Model file for the job. Use its own axes, mm. Face numbers are marked on the shaded views. Coordinates: 2 decimals unless noted, no trailing zeros. Order: outer loops, then holes, each group sorted by start corner. A loop starts at its lowest first (then second) coordinate and runs counter-clockwise, first axis right, second up. Notation, with made-up numbers: (21.25, -21.75) -> (51.25, -21.75) arc R27 ccw to (51.25, 10.25) -> close; hole circle Ø9 at (-37, 38.5). An arc over 180 degrees is marked (long way). Use CSV: the item, a comma, the result in double quotes. Start each with the question number.
(1) Cut at A-A on x = 0. Write the cut outline in (y, z), plus the area to 3 significant figures.
(2) Cut at B-B on z = 0. Write the cut outline in (x, y).
(3) Cut at C-C on y = 0.25. Write the cut outline in (x, z), plus the area to 3 significant figures.
(4) Probe L1, parallel to X at y = -1.7, z = 0; L2, parallel to X at y = 1.5, z = -2.25; L3, parallel to Z at x = -0.75, y = -1.5. List the from-to ranges inside material, lowest first.
(5) Pin check, flat tip, straight feed: pin 1 Ø1.5 at (x, y) = (-1, 0) entering from -Z. Stop position of the tip, or through.
(6) Pull direction Z, two halves, no side cores. Call the marked faces 1, 2 and 3: pulls with the +Z half, pulls with the -Z half, needs draft (parallel to the pull), parting line crosses it, or undercut.
```python
from build123d import *

# Parameters (mm, degrees)
SKETCH1_R           = 11
SKETCH1_R_2         = 4
BOSS_EXTRUDE1_DEPTH = 3.5
FILLET1_R           = 1.5
FILLET2_R           = 0.5


with BuildPart() as part:
    # Sketch1 → Boss-Extrude1 (new body, symmetric)
    with BuildSketch(Plane(origin=(0, 0, 0), x_dir=(1, 0, 0), z_dir=(0, 1, 0))):
        with Locations(Location((0, 0, 0), (0, 0, 270))):  # turned: the seam where the file's is
            Circle(SKETCH1_R)
        with Locations(Location((0, 0, 0), (0, 0, 270))):  # turned: the seam where the file's is
            Circle(SKETCH1_R_2, mode=Mode.SUBTRACT)
    extrude(amount=BOSS_EXTRUDE1_DEPTH, both=True)

    # Fillet1
    fillet1_edges = [part.edges().sort_by_distance(p)[0] for p in [
        (0, -3.5, -11),
        (0, 3.5, -11),
    ]]
    fillet(fillet1_edges, radius=FILLET1_R)

    # Fillet2
    fillet2_edges = [part.edges().sort_by_distance(p)[0] for p in [
        (0, -3.5, -4),
        (0, 3.5, -4),
    ]]
    fillet(fillet2_edges, radius=FILLET2_R)


solid = part.part
```
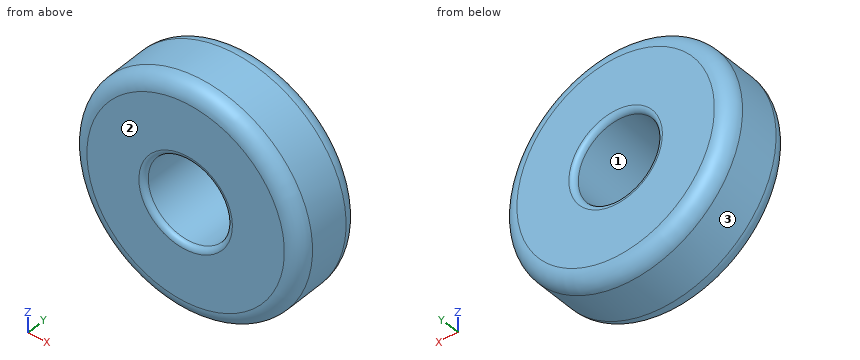
Outcome:
1,outline,"(-3.5, -9.5) arc R1.5 ccw to (-2, -11) -> (2, -11) arc R1.5 ccw to (3.5, -9.5) -> (3.5, -4.5) arc R0.5 ccw to (3, -4) -> (-3, -4) arc R0.5 ccw to (-3.5, -4.5) -> close; (-3.5, 4.5) arc R0.5 ccw to (-3, 4) -> (3, 4) arc R0.5 ccw to (3.5, 4.5) -> (3.5, 9.5) arc R1.5 ccw to (2, 11) -> (-2, 11) arc R1.5 ccw to (-3.5, 9.5) -> close"
1,area,"95.9 mm2"
2,outline,"(-11, -2) arc R1.5 ccw to (-9.5, -3.5) -> (-4.5, -3.5) arc R0.5 ccw to (-4, -3) -> (-4, 3) arc R0.5 ccw to (-4.5, 3.5) -> (-9.5, 3.5) arc R1.5 ccw to (-11, 2) -> close; (4, -3) arc R0.5 ccw to (4.5, -3.5) -> (9.5, -3.5) arc R1.5 ccw to (11, -2) -> (11, 2) arc R1.5 ccw to (9.5, 3.5) -> (4.5, 3.5) arc R0.5 ccw to (4, 3) -> close"
3,outline,"circle Ø22 at (0, 0); hole circle Ø8 at (0, 0)"
3,area,"330 mm2"
4,L1,"-11 to -4, 4 to 11"
4,L2,"-10.77 to -3.31, 3.31 to 10.77"
4,L3,"-10.97 to -3.93, 3.93 to 10.97"
5,pin 1,"z = -11"
6,face 1,"undercut"
6,face 2,"needs draft"
6,face 3,"parting line crosses it"
